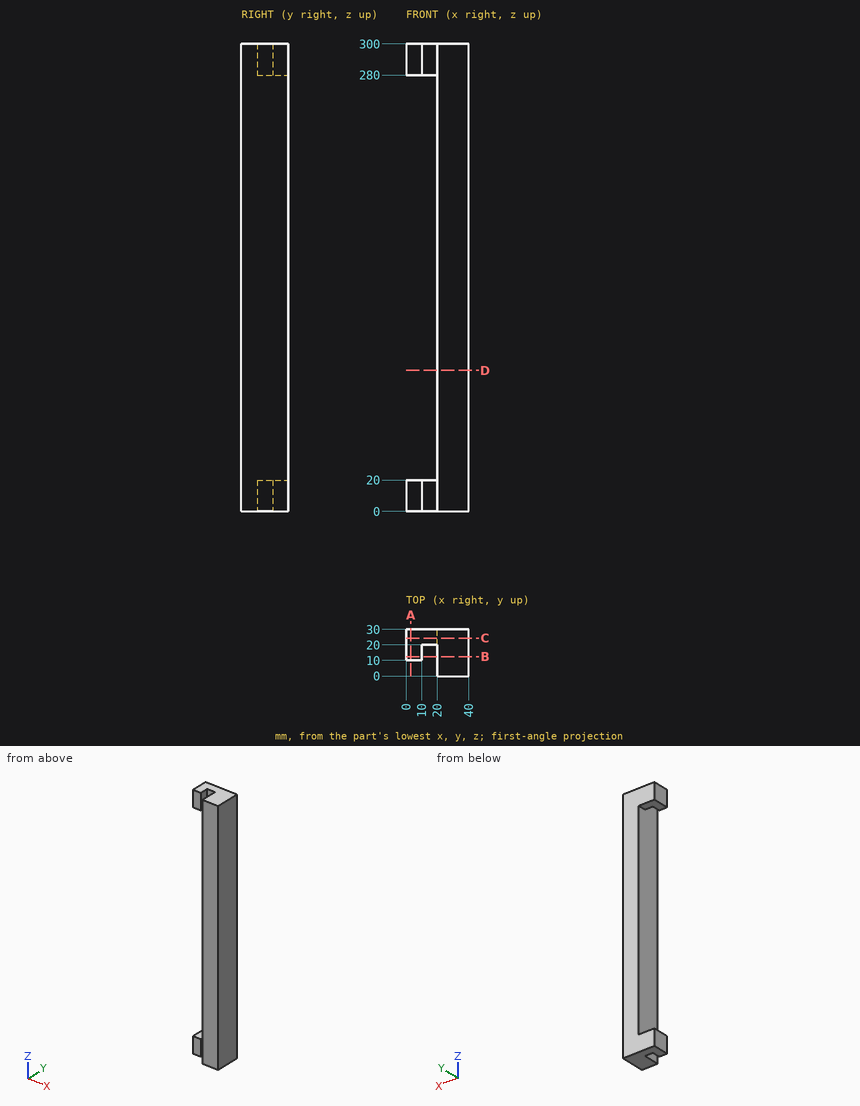
The figure shows three views and two pictorial views of one solid part (mm, origin at its lowest corner). Answer the questions. Round coordinates to 2 decimals unless told otherwise and drop trailing zeros. Order: outer loops, then holes, each group sorted by start corner. A loop starts at its lowest first (then second) coordinate and runs counter-clockwise, first axis right, second up. Notation, with made-up numbers: M 85.5,17.5 L 113.5,17.5 A19 cw 113.5,24.5 Z; hole C 24.25,18.5 d10. An arc over 180 degrees is marked long. Put each result on its own line as item: value. Start each with the question number.
Q1. Section C-C, the plane y = 24.25 is taken. Write down the section's boundary in (x, z).
Q2. Flat-ended cylindrical pins translate along their axes: pin 1 (3 mm diameter, centred on x = 14.5, z = 286, fed in from -Y); pin 2 (11 mm diameter, centred on x = 2.5, z = 13, fed in from -Y); pin 3 (3 mm diameter, centred on x = 27, z = 262, fed in from -Y); pin 4 (9 mm diameter, centred on y = 12.5, z = 157.5, fed in from -X). Find the tip coordinate at first contact, or state that the pin passes through.
Q3. Straight lines are drawn through the part: L1, parallel to Z at x = 7, y = 20; L2, parallel to X at y = 2.5, z = 170. For each, find the intervals that lie inside material, in ascending order. Write a range as [from, to].
Q4. Section A-A, the plane x = 3 is taken. Write down the section's boundary in (y, z).
Q5. Section D-D, the plane z = 90.5 is taken. Write down the section's boundary in (x, y), and give its area (3 significant figures).
Q6. Section B-B, the plane y = 12.5 is taken. Write down the section's boundary in (x, z).
Findings below:
1. outline: M 0,0 L 40,0 L 40,300 L 0,300 L 0,280 L 20,280 L 20,20 L 0,20 Z
2. pin 1: stops at y = 20
2. pin 2: stops at y = 10
2. pin 3: stops at y = 0
2. pin 4: stops at x = 20
3. L1: z = [0, 20], [280, 300]
3. L2: x = [20, 40]
4. outline: M 10,0 L 30,0 L 30,20 L 10,20 Z; M 10,280 L 30,280 L 30,300 L 10,300 Z
5. outline: M 20,0 L 40,0 L 40,30 L 20,30 Z
5. area: 600 mm^2
6. outline: M 0,0 L 10,0 L 10,20 L 0,20 Z; M 0,280 L 10,280 L 10,300 L 0,300 Z; M 20,0 L 40,0 L 40,300 L 20,300 Z
